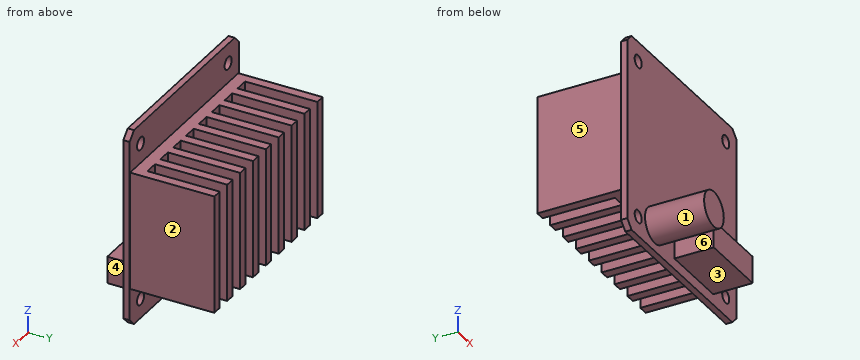
```python
from build123d import *

# Parameters (mm, degrees)
SKETCH1_R                = 1.6
BOSS_EXTRUDE1_DEPTH      = 1.6
BOSS_EXTRUDE2_DEPTH      = 15
BOSS_EXTRUDE2_DEPTH_BACK = 15
SKETCH3_R                = 4.484115481
BOSS_EXTRUDE3_DEPTH      = 15
SKETCH4_W                = 17.802607731
SKETCH4_H                = 6.826563867
BOSS_EXTRUDE4_DEPTH      = 10


with BuildPart() as part:
    # Sketch1 → Boss-Extrude1 (new body)
    with BuildSketch(Plane(origin=(0, 0, 0), x_dir=(1, 0, 0), z_dir=(0, 1, 0))):
        Polygon((-25, 23), (-23, 25), (23, 25), (25, 23), (25, -23), (23, -25), (-23, -25), (-25, -23), align=None)
        with Locations((20, 20)):
            Circle(SKETCH1_R, mode=Mode.SUBTRACT)
        with Locations((-20, 20)):
            Circle(SKETCH1_R, mode=Mode.SUBTRACT)
        with Locations((-20, -20)):
            Circle(SKETCH1_R, mode=Mode.SUBTRACT)
        with Locations((20, -20)):
            Circle(SKETCH1_R, mode=Mode.SUBTRACT)
    extrude(amount=BOSS_EXTRUDE1_DEPTH)

    # Sketch2 → Boss-Extrude2 (add, two sides)
    with BuildSketch(Plane.XY) as boss_extrude2_sk:
        Polygon((-24.671549394, 1.6), (-24.671549394, 23.015646785), (-22.237958156, 23.015646785), (-22.237958156, 4.666777426), (-18.788248299, 4.666777426), (-18.788248299, 23.015646785), (-16.354657061, 23.015646785), (-16.354657061, 4.666777426), (-12.904947204, 4.666777426), (-12.904947204, 23.015646785), (-10.471355966, 23.015646785), (-10.471355966, 4.666777426), (-7.021646108, 4.666777426), (-7.021646108, 23.015646785), (-4.588054871, 23.015646785), (-4.588054871, 4.666777426), (-1.138345013, 4.666777426), (-1.138345013, 23.015646785), (1.295246225, 23.015646785), (1.295246225, 4.666777426), (4.744956082, 4.666777426), (4.744956082, 23.015646785), (7.17854732, 23.015646785), (7.17854732, 4.666777426), (10.628257178, 4.666777426), (10.628257178, 23.015646785), (13.061848415, 23.015646785), (13.061848415, 4.666777426), (16.511558273, 4.666777426), (16.511558273, 23.015646785), (18.945149511, 23.015646785), (18.945149511, 4.666777426), (22.394859368, 4.666777426), (22.394859368, 23.015646785), (24.828450606, 23.015646785), (24.828450606, 1.6), align=None)
    extrude(amount=BOSS_EXTRUDE2_DEPTH)
    extrude(boss_extrude2_sk.sketch, amount=-BOSS_EXTRUDE2_DEPTH_BACK)

    # Sketch3 → Boss-Extrude3 (add)
    with BuildSketch(Plane.XZ):
        with Locations((-12.381512895, -18.471878698)):
            Circle(SKETCH3_R)
    extrude(amount=BOSS_EXTRUDE3_DEPTH)

    # Sketch4 → Boss-Extrude4 (add)
    with BuildSketch(Plane.XZ):
        with Locations((5.421094835, -18.873441279)):
            Rectangle(SKETCH4_W, SKETCH4_H)
    extrude(amount=BOSS_EXTRUDE4_DEPTH)


solid = part.part
```
CAD build for the part. Positions are in the model's coordinates, mm. Face numbers are marked on the shaded views. A direction names the side the tool comes from. Coordinates: 2 decimals unless noted, no trailing zeros. Write each loop counter-clockwise with the first axis right and the second up, starting at its lowest first coordinate (ties: lowest second). Pieces come first, ordered by that corner, then holes.
(1) Two-plate mould, pull along X, no slides. Class the marked faces 1, 2 and 3: +X half, -X half, draft (parallel to the pull), parting line (faces both ways), or undercut.
(2) 3-axis set-ups, long thin cutter, end or side, ignore diameter. For the marked faces 4, 5 and 6: which of +Z, -Z, +X, -X, +Y, -Y reach the whole face in a straight line?
(3) Cut at C-C, the plane x = 6. List the corners of the cut face in (y, z).
(4) Cut at A-A, the plane z = 20. List the corners of the cut face in (x, y), and give its area (3 significant figures).
(5) Flat gauge pins, fed straight in: pin 1 (5 mm diameter, centred on x = 20, z = -20, fed in from +Y); pin 2 (5.5 mm diameter, centred on y = 17, z = -5, fed in from +X); pin 3 (15 mm diameter, centred on x = -3, z = 0.5, fed in from -Y). Where does each tip first touch, or does it go through?
(6) Drill centre lines: probe 1 along Z at (x, y) = (-20, 1); probe 2 along Y at (x, z) = (6.5, 9). Where is each one in solid material? Low to high.
(7) Cut at B-B, the plane x = -20. List the corners of the cut face in (y, z), and give its area (3 significant figures).
(8) Cut at D-D, the plane y = 3.5. List the corners of the cut face in (x, z).
Geometry says:
1. face 1: undercut
1. face 2: +X half
1. face 3: draft
2. face 4: +Z, -Z, +X, -Y
2. face 5: +Z, -Z, -X, +Y
2. face 6: +Z, -Z, -Y
3. outline: (-10, -22.29) - (0, -22.29) - (0, -25) - (1.6, -25) - (1.6, -15) - (23.02, -15) - (23.02, 15) - (1.6, 15) - (1.6, 25) - (0, 25) - (0, -15.46) - (-10, -15.46) - close
4. outline: (-25, 0) - (-21.6, 0) - (-21.6, 1.6) - (-25, 1.6) - close; (-18.4, 0) - (18.4, 0) - (18.4, 1.6) - (-18.4, 1.6) - close; (21.6, 0) - (25, 0) - (25, 1.6) - (21.6, 1.6) - close
4. area: 69.8 mm2
5. pin 1: stops at y = 1.6
5. pin 2: stops at x = 24.83
5. pin 3: stops at y = 0
6. probe 1: z = -25 to -21.6, -18.4 to 18.4, 21.6 to 25
6. probe 2: y = 0 to 23.02
7. outline: (0, -25) - (1.6, -25) - (1.6, -21.6) - (0, -21.6) - close; (0, -18.4) - (1.6, -18.4) - (1.6, -15) - (4.67, -15) - (4.67, 15) - (1.6, 15) - (1.6, 18.4) - (0, 18.4) - close; (0, 21.6) - (1.6, 21.6) - (1.6, 25) - (0, 25) - close
7. area: 162 mm2
8. outline: (-24.67, -15) - (24.83, -15) - (24.83, 15) - (-24.67, 15) - close
